Check sheet for the modelled part. Datum: model origin and axes. Units: mm. A direction names the side the tool comes from. Round coordinates to 2 decimals unless told otherwise and drop trailing zeros. Order: outer loops, then holes, each group sorted by start corner. A loop starts at its lowest first (then second) coordinate and runs counter-clockwise, first axis right, second up.
```python
from build123d import *

# Parameters (mm, degrees)
CUT_EXTRUDE2_REACH      = 152.804
CUT_EXTRUDE2_END_RADIUS = 57.15
SKETCH3_R               = 3.175
CIRPATTERN2_COUNT       = 8


with BuildPart() as part:
    # Sketch1 → Revolve2 (revolve)
    with BuildSketch(Plane.XY, mode=Mode.PRIVATE) as revolve2_sk:
        with BuildLine():
            Line((6.35, 45.363399312), (6.35, 32.663399312))
            ThreePointArc((6.35, 32.663399312), (27.556037661, 22.529619114), (50.8, 19.05))
            Line((50.8, 19.05), (63.5, 19.05))
            Line((63.5, 19.05), (63.5, 22.225))
            Line((63.5, 22.225), (60.325, 22.225))
            Line((60.325, 22.225), (60.325, 25.4))
            Line((60.325, 25.4), (63.5, 25.4))
            Line((63.5, 25.4), (63.5, 28.575))
            Line((63.5, 28.575), (60.325, 28.575))
            Line((60.325, 28.575), (60.325, 31.75))
            Line((60.325, 31.75), (63.5, 31.75))
            Line((63.5, 31.75), (63.5, 50.8))
            Line((63.5, 50.8), (57.15, 50.8))
            Line((57.15, 50.8), (57.15, 25.4))
            Line((57.15, 25.4), (12.7, 39.013399312))
            Line((12.7, 39.013399312), (12.7, 45.363399312))
            Line((12.7, 45.363399312), (6.35, 45.363399312))
        make_face()
    revolve(revolve2_sk.sketch.rotate(Axis((0, 0, 0), (0, 1, 0)), 90), axis=Axis((0, 0, 0), (0, 1, 0)))

    # Cut-Extrude2: up to this cylinder (the profile starts outside it)
    cut_extrude2_end = Plane(origin=(0, 38.1, 0), z_dir=(0, -1, 0)) * Cylinder(CUT_EXTRUDE2_END_RADIUS, 420.908, mode=Mode.PRIVATE)
    # Sketch3 → Cut-Extrude2 (cut, up to the surface)
    with BuildSketch(Plane.XY.offset(63.5), mode=Mode.PRIVATE) as cut_extrude2_sk1:
        with Locations((0, 38.1)):
            Circle(SKETCH3_R)
    cut_extrude2_tool1 = extrude(cut_extrude2_sk1.sketch, amount=-CUT_EXTRUDE2_REACH, mode=Mode.PRIVATE) - cut_extrude2_end
    cut_extrude2 = cut_extrude2_tool1.solids().sort_by_distance((0, 38.1, 63.5))[0]
    add(cut_extrude2, mode=Mode.SUBTRACT)

    # CirPattern2: Cut-Extrude2 ×8 about axis
    cirpattern2_axis = Axis((0, 0, 0), (0, -1, 0))
    for i in range(1, CIRPATTERN2_COUNT):
        add(cut_extrude2.rotate(cirpattern2_axis, i * 360 / CIRPATTERN2_COUNT), mode=Mode.SUBTRACT)


solid = part.part
```
Item 1: Access from +Z, -Z, +X, -X, +Y, -Y to the whole of each face (thin tool, end or side, straight path). Record for faces 1 (the flat face through (23, 28.575, -56)), 2 (the cylindrical face through (-60.33, 35, -0.69)), 3 (the cylindrical face through (60.33, 35, 0.69)), 4 (the cylindrical face through (21.89, 37.92, -52.79)), 5 (the cylindrical face through (-0.69, 35, 60.33)).
Answer:
face 1: none
face 2: -X
face 3: +X
face 4: +Y
face 5: +Z
Item 2: Scan lines: line 1 along Y through (x, z) = (-62, 0) (3 decimals); line 2 along Z through (x, y) = (1.5, 47); line 3 along Y through (x, z) = (0, 60) (3 decimals). Record each from-to range of solid material in increasing order.
Answer:
line 1: y = 19.05 to 22.225, 25.4 to 28.575, 31.75 to 34.925, 41.275 to 50.8
line 2: z = -63.48 to -57.13, 57.13 to 63.48
line 3: y = 19.05 to 34.925, 41.275 to 50.8
Item 3: Go/stop test with flat-tipped pins: P1, Ø1.5, axis at x = -2.5, y = 42.5, coming from the -Z side; P2, Ø10, axis at x = -7, z = 39, coming from the -Y side; P3, Ø4, axis at x = -42.5, y = 29.5, coming from the -Z side. Record where each tip stops, or that it passes through.
Answer:
P1: stops at z = -63.48
P2: stops at y = 19.29
P3: stops at z = -48.72
Item 4: Sectioned sample at C-C (y = 47.5). Record the cut outline in (x, z), and give its area (3 significant figures).
Answer:
outline: circle Ø127 at (0, 0); hole circle Ø114.3 at (0, 0)
area: 2,410 mm2
Item 5: Sectioned sample at A-A (z = 0). State how many separate pieces and enclosed holes the cut face has, and give its area (3 significant figures).
Answer:
separate pieces: 4
enclosed holes: 0
area: 1,400 mm2
Item 6: Release check for a two-part mould opening along Z. For faces 6 (the cylindrical face through (-2.652, 23.835, 60.267)), 7 (the cylindrical face through (7.7, 42.2, 10.1)), 8 (the flat face through (23, 22.225, -56)) record: released by +Z, released by -Z, zero draft, split by the parting line, or undercut.
Answer:
face 6: split by the parting line
face 7: undercut
face 8: zero draft
